```python
from build123d import *

# Parameters (mm, degrees)
SKETCH2_W           = 478
SKETCH2_H           = 809.900101531
SKETCH2_R           = 3.175
SKETCH2_R_2         = 3.96875
BOSS_EXTRUDE1_DEPTH = 1.6002


with BuildPart() as part:
    # Sketch2 → Boss-Extrude1 (new body)
    with BuildSketch(Plane.XY):
        with Locations((-130.152406859, 514.031343345)):
            Rectangle(SKETCH2_W, SKETCH2_H)
        with Locations((-362.710206859, 115.522426029)):
            Circle(SKETCH2_R, mode=Mode.SUBTRACT)
        with Locations((102.405393141, 912.54036211)):
            Circle(SKETCH2_R, mode=Mode.SUBTRACT)
        with Locations((-362.710206859, 912.54036211)):
            Circle(SKETCH2_R, mode=Mode.SUBTRACT)
        with Locations((102.405393141, 115.522426029)):
            Circle(SKETCH2_R, mode=Mode.SUBTRACT)
        with Locations((86.893613141, 514.031343345)):
            Circle(SKETCH2_R_2, mode=Mode.SUBTRACT)
        with Locations((-347.198426859, 514.031343345)):
            Circle(SKETCH2_R_2, mode=Mode.SUBTRACT)
        Polygon((63.111393141, 112.35889233), (63.111393141, 229.898149855), (63.111393141, 268.081394028), (58.348893141, 268.081394028), (58.348893141, 229.898149855), (-318.667460794, 229.898149855), (-318.667460794, 268.081394028), (-323.429960794, 268.081394028), (-323.429960794, 229.898149855), (-323.429960794, 112.35889233), (-318.667460794, 112.35889233), (-318.667460794, 138.081394028), (58.348893141, 138.081394028), (58.348893141, 112.35889233), align=None, mode=Mode.SUBTRACT)
    extrude(amount=BOSS_EXTRUDE1_DEPTH)


solid = part.part
```
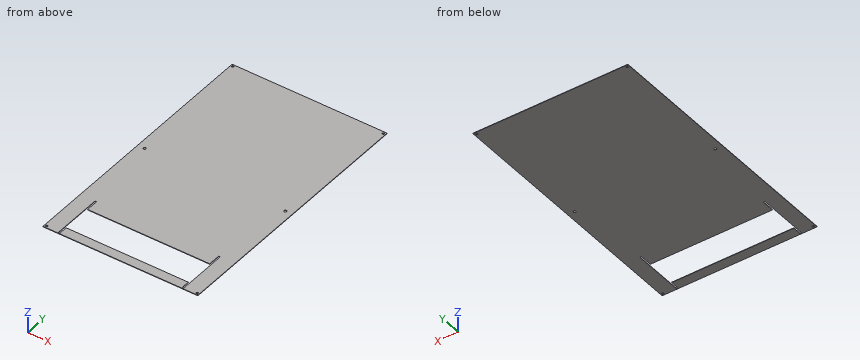
Input: part model. Units: mm. Frame: model coordinates. Coordinates: 2 decimals unless noted, no trailing zeros. Order: outer loops, then holes, each group sorted by start corner. A loop starts at its lowest first (then second) coordinate and runs counter-clockwise, first axis right, second up. Notation, with made-up numbers: (45, 57.25) - (57, 57.25) arc R28 cw to (57, 93.25) - close; hole circle Ø5 at (-6, 34). An arc over 180 degrees is marked (long way). Put each result on its own line as item: value.
1. Cut plane C-C on z = 0.8. State how many separate pieces and enclosed holes the cut face has, then the cut area to 3 significant figures.
Report:
separate pieces: 1
enclosed holes: 7
area: 351,000 mm2
2. Cut plane B-B on x = -6. Return the cut outline in (y, z), then the cut area to 3 significant figures.
Report:
outline: (109.08, 0) - (138.08, 0) - (138.08, 1.6) - (109.08, 1.6) - close; (229.9, 0) - (918.98, 0) - (918.98, 1.6) - (229.9, 1.6) - close
area: 1,150 mm2
3. Line query: line 1 along Y through (x, z) = (-174, 0.1); line 2 along X through (y, z) = (242, 0.65); line 3 along X through (y, z) = (182, 0.5). Output: solid intervals per line, ascending.
Report:
line 1: y = 109.08 to 138.08, 229.9 to 918.98
line 2: x = -369.15 to -323.43, -318.67 to 58.35, 63.11 to 108.85
line 3: x = -369.15 to -323.43, 63.11 to 108.85
4. Contact query for flat-ended pins moving along their axis: pin 1 Ø8.5 at (x, y) = (-362.71, 912.54) entering from -Z; pin 2 Ø6.5 at (x, y) = (-347.2, 514.03) entering from -Z. Output: stop coordinate, or through.
Report:
pin 1: stops at z = 0
pin 2: passes through
5. Cut plane A-A on y = 185. Return the cut outline in (x, z).
Report:
outline: (-369.15, 0) - (-323.43, 0) - (-323.43, 1.6) - (-369.15, 1.6) - close; (63.11, 0) - (108.85, 0) - (108.85, 1.6) - (63.11, 1.6) - close
